from build123d import *

# Parameters (mm, degrees)
SKETCH_1_W          = 6.2
SKETCH_1_H          = 6.2
SKETCH_1_R          = 1.2
EXTRUDE_1_DEPTH     = 2
CUT_EXTRUDE_1_DEPTH = 1
SKETCH_3_W          = 10
SKETCH_3_H          = 12.5
CUT_EXTRUDE_2_DEPTH = 1
SKETCH_4_W          = 44.4
SKETCH_4_H          = 18.5
SKETCH_4_W_2        = 38.4
SKETCH_4_H_2        = 12.5
EXTRUDE_2_DEPTH     = 3
CHAMFER_2_SIZE      = 2
SKETCH_5_W          = 6.2
SKETCH_5_H          = 6.2
EXTRUDE_3_DEPTH     = 2
CUT_EXTRUDE_3_DEPTH = 10
EXTRUDE_4_DEPTH     = 2
SKETCH_8_R          = 1.9
CUT_EXTRUDE_4_DEPTH = 10


with BuildPart() as part:
    # 草图1 → 凸台-拉伸1 (new body)
    with BuildSketch(Plane.XY):
        Polygon((-68.63, 16.2), (-64.63, 12.2), (-64.63, -37.62), (-68.63, -41.62), (-68.63, -49.62), (11.17, -49.62), (11.17, -41.62), (7.17, -37.62), (7.17, 12.2), (11.17, 16.2), (11.17, 38.1), (-68.63, 38.1), align=None)
        with Locations((-37.93, 28.38)):
            Rectangle(SKETCH_1_W, SKETCH_1_H, mode=Mode.SUBTRACT)
        with Locations((-27.73, 28.38)):
            Rectangle(SKETCH_1_W, SKETCH_1_H, mode=Mode.SUBTRACT)
        with Locations((-66.63, -45.62)):
            Circle(SKETCH_1_R, mode=Mode.SUBTRACT)
        with Locations((9.17, -45.62)):
            Circle(SKETCH_1_R, mode=Mode.SUBTRACT)
        with Locations((-66.63, 20.2)):
            Circle(SKETCH_1_R, mode=Mode.SUBTRACT)
        with Locations((9.17, 20.2)):
            Circle(SKETCH_1_R, mode=Mode.SUBTRACT)
    extrude(amount=EXTRUDE_1_DEPTH)

    # 草图2 → 切除-拉伸1 (cut)
    with BuildSketch(Plane.XY.offset(2)):
        Polygon((-12.23, -27.12), (-39.83, -27.12), (-39.83, -35.02), (-39.83, -39.62), (-12.23, -39.62), align=None)
        Polygon((-39.83, -27.12), (-50.63, -27.12), (-50.63, -39.62), (-39.83, -39.62), (-39.83, -35.02), align=None)
    extrude(amount=-CUT_EXTRUDE_1_DEPTH, mode=Mode.SUBTRACT)

    # 草图3 → 切除-拉伸2 (cut)
    with BuildSketch(Plane.XY.offset(1)):
        with Locations((-45.63, -33.37)):
            Rectangle(SKETCH_3_W, SKETCH_3_H)
    extrude(amount=-CUT_EXTRUDE_2_DEPTH, mode=Mode.SUBTRACT)

    # 草图4 → 凸台-拉伸2 (add)
    with BuildSketch(Plane.XY.offset(2)):
        with Locations((-31.43, -33.37)):
            Rectangle(SKETCH_4_W, SKETCH_4_H)
        with Locations((-31.43, -33.37)):
            Rectangle(SKETCH_4_W_2, SKETCH_4_H_2, mode=Mode.SUBTRACT)
    extrude(amount=EXTRUDE_2_DEPTH)

    # 倒角2
    chamfer_2_edges = [part.edges().sort_by_distance(p)[0] for p in [
        (-31.43, -24.12, 5),
        (-9.23, -33.37, 5),
        (-53.63, -33.37, 5),
        (-31.43, -42.62, 5),
    ]]
    chamfer(chamfer_2_edges, length=CHAMFER_2_SIZE)

    # 草图5 → 凸台-拉伸3 (add)
    with BuildSketch(Plane.XY.offset(2)):
        with Locations((-37.93, 28.38)):
            Rectangle(SKETCH_5_W, SKETCH_5_H)
        with Locations((-27.73, 28.38)):
            Rectangle(SKETCH_5_W, SKETCH_5_H)
    extrude(amount=-EXTRUDE_3_DEPTH)

    # 草图6 → 切除-拉伸3 (cut)
    with BuildSketch(Plane.XY.offset(2)):
        with BuildLine():
            Line((-37.73, 30.5), (-37.73, 29.1))
            Line((-37.73, 29.1), (-36.33, 29.1))
            ThreePointArc((-36.33, 29.1), (-36.740050506, 30.089949494), (-37.73, 30.5))
        make_face()
        with BuildLine():
            Line((-36.33, 29.1), (-37.73, 29.1))
            Line((-37.73, 29.1), (-37.73, 30.5))
            ThreePointArc((-37.73, 30.5), (-38.719949494, 28.110050506), (-36.33, 29.1))
        make_face()
        with BuildLine():
            ThreePointArc((-19.73, 30.5), (-20.719949494, 30.089949494), (-21.13, 29.1))
            Line((-21.13, 29.1), (-19.73, 29.1))
            Line((-19.73, 29.1), (-19.73, 30.5))
        make_face()
        with BuildLine():
            Line((-19.73, 29.1), (-21.13, 29.1))
            ThreePointArc((-21.13, 29.1), (-19.73, 27.7), (-18.33, 29.1))
            ThreePointArc((-18.33, 29.1), (-18.740050506, 30.089949494), (-19.73, 30.5))
            Line((-19.73, 30.5), (-19.73, 29.1))
        make_face()
    extrude(amount=-CUT_EXTRUDE_3_DEPTH, mode=Mode.SUBTRACT)

    # 草图7 → 凸台-拉伸4 (add)
    with BuildSketch(Plane.XY.offset(2)):
        Polygon((-68.63, 38.1), (-74.61, 38.1), (-74.61, -41.62), (-68.63, -41.62), (-64.63, -37.62), (-64.63, 12.2), (-68.63, 16.2), align=None)
        Polygon((17.15, 38.1), (11.17, 38.1), (11.17, 16.2), (7.17, 12.2), (7.17, -37.62), (11.17, -41.62), (17.15, -41.62), align=None)
        Polygon((11.17, -41.62), (11.17, -49.62), (17.15, -41.62), align=None)
        Polygon((-68.63, -41.62), (-74.61, -41.62), (-68.63, -49.62), align=None)
    extrude(amount=-EXTRUDE_4_DEPTH)

    # 草图8 → 切除-拉伸4 (cut)
    with BuildSketch(Plane(origin=(0, 0, 0), x_dir=(-1, 0, 0), z_dir=(0, 0, -1))):
        with Locations((66.61, -11.746314383)):
            Circle(SKETCH_8_R)
        with Locations((-9.156491604, -11.746314383)):
            Circle(SKETCH_8_R)
    extrude(amount=-CUT_EXTRUDE_4_DEPTH, mode=Mode.SUBTRACT)


solid = part.part
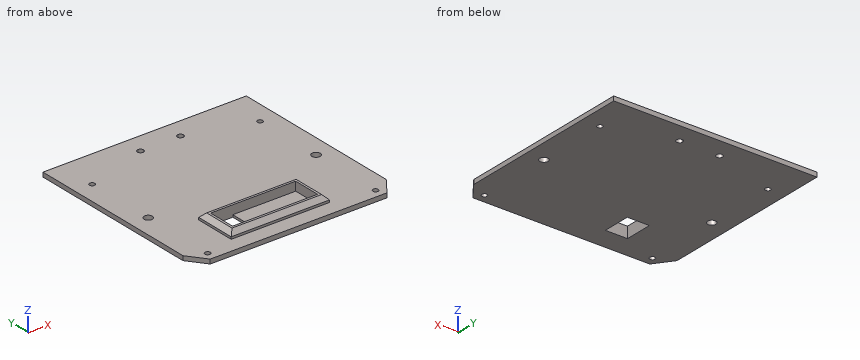
Here's how the part is built. I have some questions about the finished solid (model axes, mm). Round coordinates to 2 decimals unless told otherwise and drop trailing zeros. Order: outer loops, then holes, each group sorted by start corner. A loop starts at its lowest first (then second) coordinate and runs counter-clockwise, first axis right, second up. Notation, with made-up numbers: (-21.75, 79.25) -> (28.25, 79.25) arc R16 cw to (28.25, 109.25) -> close; hole circle Ø10 at (17, 25). An arc over 180 degrees is marked (long way). Return JSON: item names as keys, results as strings.
Q1. I need wall thicknesses on line 1 along Y through (x, z) = (-66.61, 1.15); line 2 along Y through (x, z) = (-34.5, 1.6); line 3 along Z through (x, y) = (-11.5, 2). Which ranges of each line are inside material? Lowest first, please. Write a range as from..to.
Filled sheet:
{"line 1": "y = -49.62..-46.82, -44.42..-13.65, -9.85..19, 21.4..38.1", "line 2": "y = -49.62..-39.62, -27.12..38.1", "line 3": "z = 0..2"}
Q2. For pin 1 Ø0.5 at (y, z) = (-31, 2.5) entering from -X; pin 2 Ø5 at (x, y) = (-2, -28.5) entering from +Z; pin 3 Ø0.8 at (x, z) = (-23, 2.5) entering from -Y, each with a flat end and sliding along its axis, tell me the tip position at first contact or that it passes through.
Filled sheet:
{"pin 1": "stops at x = -53.63", "pin 2": "stops at z = 2", "pin 3": "stops at y = -42.62"}
Q3. If we section it at C-C on x = -46: List the corners of the cut face in (y, z) for me.
Filled sheet:
{"outline": "(-49.62, 0) -> (-39.62, 0) -> (-39.62, 5) -> (-40.62, 5) -> (-42.62, 3) -> (-42.62, 2) -> (-49.62, 2) -> close; (-27.12, 0) -> (38.1, 0) -> (38.1, 2) -> (-24.12, 2) -> (-24.12, 3) -> (-26.12, 5) -> (-27.12, 5) -> close"}
Q4. If we section it at D-D on x = -30: List the corners of the cut face in (y, z) for me.
Filled sheet:
{"outline": "(-49.62, 0) -> (38.1, 0) -> (38.1, 2) -> (-24.12, 2) -> (-24.12, 3) -> (-26.12, 5) -> (-27.12, 5) -> (-27.12, 1) -> (-39.62, 1) -> (-39.62, 5) -> (-40.62, 5) -> (-42.62, 3) -> (-42.62, 2) -> (-49.62, 2) -> close"}
Q5. If we section it at B-B on z = 3.9: List the corners of the cut face in (x, y) for me, plus the area to 3 significant figures.
Filled sheet:
{"outline": "(-52.73, -41.72) -> (-10.13, -41.72) -> (-10.13, -25.02) -> (-52.73, -25.02) -> close; hole (-50.63, -39.62) -> (-12.23, -39.62) -> (-12.23, -27.12) -> (-50.63, -27.12) -> close", "area": "231 mm^2"}
Q6. If we section it at A-A on y = -45.62: List the corners of the cut face in (x, z) for me.
Filled sheet:
{"outline": "(-71.62, 0) -> (-67.83, 0) -> (-67.83, 2) -> (-71.62, 2) -> close; (-65.43, 0) -> (7.97, 0) -> (7.97, 2) -> (-65.43, 2) -> close; (10.37, 0) -> (14.16, 0) -> (14.16, 2) -> (10.37, 2) -> close"}
